Source: CAD feature listing. Evaluate the final solid. Frame: model axes, mm. A direction names the side the tool comes from. Give positions to 0.01 mm unless a question says otherwise; leave off trailing zeros. Write each loop counter-clockwise with the first axis right and the second up, starting at its lowest first coordinate (ties: lowest second). Pieces come first, ordered by that corner, then holes. Notation, with made-up numbers: M 15,25.25 L 73,25.25 A17 ccw 73,57.25 Z; hole C 14.25,67 d7. An arc over 180 degrees is marked long. Return JSON: item names as keys, results as strings.
```python
from build123d import *

# Parameters (mm, degrees)
BOSS_EXTRUDE1_DEPTH = 100
SKETCH2_R           = 5
CUT_EXTRUDE1_DEPTH  = 100
SKETCH6_W           = 44
SKETCH6_H           = 44
CUT_EXTRUDE2_DEPTH  = 11
SKETCH7_R           = 1.55
CUT_EXTRUDE3_DEPTH  = 11


with BuildPart() as part:
    # Sketch1 → Boss-Extrude1 (new body)
    with BuildSketch(Plane.XY):
        Polygon((0, 0), (0, 280), (120, 280), (120, 300), (-20, 300), (-20, 20), (-120, 20), (-120, 0), align=None)
    extrude(amount=BOSS_EXTRUDE1_DEPTH)

    # Sketch2 → Cut-Extrude1 (cut)
    with BuildSketch(Plane(origin=(0, 300, 0), x_dir=(1, 0, 0), z_dir=(0, 1, 0))):
        with Locations(Location((77.5, -50, 0), (0, 0, 270))):
            Circle(SKETCH2_R)
    extrude(amount=-CUT_EXTRUDE1_DEPTH, mode=Mode.SUBTRACT)

    # Sketch6 → Cut-Extrude2 (cut)
    with BuildSketch(Plane(origin=(0, 300, 0), x_dir=(1, 0, 0), z_dir=(0, 1, 0))):
        with Locations((77.5, -50)):
            Rectangle(SKETCH6_W, SKETCH6_H)
    extrude(amount=-CUT_EXTRUDE2_DEPTH, mode=Mode.SUBTRACT)

    # Sketch7 → Cut-Extrude3 (cut)
    with BuildSketch(Plane(origin=(0, 289, 0), x_dir=(1, 0, 0), z_dir=(0, 1, 0))):
        with Locations(Location((62, -34.5, 0), (0, 0, 270))):
            Circle(SKETCH7_R)
        with Locations(Location((93, -34.5, 0), (0, 0, 270))):
            Circle(SKETCH7_R)
        with Locations(Location((93, -65.5, 0), (0, 0, 270))):
            Circle(SKETCH7_R)
        with Locations(Location((62, -65.5, 0), (0, 0, 270))):
            Circle(SKETCH7_R)
    extrude(amount=-CUT_EXTRUDE3_DEPTH, mode=Mode.SUBTRACT)


solid = part.part
```
1) Cut plane C-C, the plane z = 12. Return the cut outline in (x, y).
Numbers:
{"outline": "M -120,0 L 0,0 L 0,280 L 120,280 L 120,300 L -20,300 L -20,20 L -120,20 Z"}
2) Set-up query: faces 4 (the face through (55.5, 295, 50)), 5 (the face through (0, 138, 49)), 6 (the face through (-69, 20, 49)). Return all of +Z, -Z, +X, -X, +Y, -Y with unobstructed straight access to the full face (end or side cutting, diameter ignored); none if empty.
Numbers:
{"face 4": "+Y", "face 5": "+Z, -Z, +X, -Y", "face 6": "+Z, -Z, -X, +Y"}
3) Contact query for flat-ended pins moving along their axis: pin 1 Ø3 at (y, z) = (242.5, 20.5) entering from +X; pin 2 Ø4 at (x, z) = (62, 34.5) entering from -Y; pin 3 Ø2.5 at (x, z) = (93, 65.5) entering from +Y; pin 4 Ø10 at (y, z) = (265, 86.5) entering from -X. Output: stop coordinate, or through.
Numbers:
{"pin 1": "stops at x = 0", "pin 2": "stops at y = 280", "pin 3": "passes through", "pin 4": "stops at x = -20"}
4) Cut plane B-B, the plane x = 77.5. Return the cut outline in (y, z), then the cut area to 3 significant figures.
Numbers:
{"outline": "M 280,0 L 300,0 L 300,28 L 289,28 L 289,45 L 280,45 Z; M 280,55 L 289,55 L 289,72 L 300,72 L 300,100 L 280,100 Z", "area": "1,430 mm²"}
5) Draft query along X for faces 1 (the face through (-20, 162, 49)), 2 (the face through (77.2, 289, 44.8)), 3 (the face through (59, 280, 49)). Return one class per face: released by +X, released by -X, zero draft, split by the parting line, or undercut.
Numbers:
{"face 1": "released by -X", "face 2": "undercut", "face 3": "zero draft"}
6) Line query: line 1 (Z direction, x = 93, y = 287); line 2 (X direction, y = 283.25, z = 34.5); line 3 (X direction, y = 282, z = 50). Output: solid intervals per line, ascending. Write a range as [from, to].
Numbers:
{"line 1": "z = [0, 32.95], [36.05, 63.95], [67.05, 100]", "line 2": "x = [-20, 60.45], [63.55, 91.45], [94.55, 120]", "line 3": "x = [-20, 72.5], [82.5, 120]"}
7) Cut plane A-A, the plane z = 50. Return the cut outline in (x, y), then the cut area to 3 significant figures.
Numbers:
{"outline": "M -120,0 L 0,0 L 0,280 L 72.5,280 L 72.5,289 L 55.5,289 L 55.5,300 L -20,300 L -20,20 L -120,20 Z; M 82.5,280 L 120,280 L 120,300 L 99.5,300 L 99.5,289 L 82.5,289 Z", "area": "9,830 mm²"}
8) Cut plane D-D, the plane y = 257. Return the cut outline in (x, z).
Numbers:
{"outline": "M -20,0 L 0,0 L 0,100 L -20,100 Z"}
